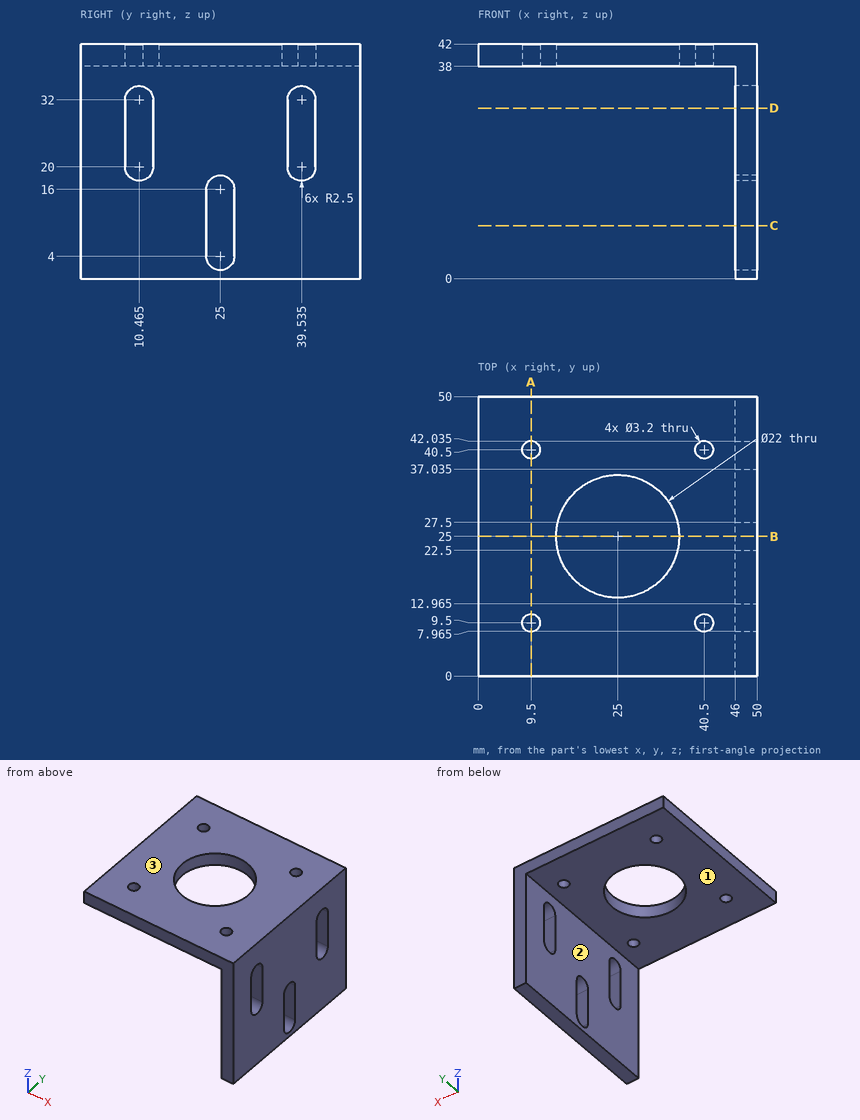
Source: three-view drawing plus pictorial views. Frame: mm from the lowest corner of the part. Coordinates: 2 decimals unless noted, no trailing zeros. Write each loop counter-clockwise with the first axis right and the second up, starting at its lowest first coordinate (ties: lowest second). Pieces come first, ordered by that corner, then holes. Notation, with made-up numbers: (77.5, 84.5) - (87.5, 84.5) arc R14 cw to (87.5, 104.5) - close; hole circle Ø9 at (-38.75, 57.25). An arc over 180 degrees is marked (long way). Return JSON: item names as keys, results as strings.
Item 1: Section query C-C (z = 9.5). Output: boundary loops of the cut face in (x, y), and give its area (3 significant figures).
Completed:
{"outline": "(46, 0) - (50, 0) - (50, 22.5) - (46, 22.5) - close; (46, 27.5) - (50, 27.5) - (50, 50) - (46, 50) - close", "area": "180 mm2"}
Item 2: Section query A-A (x = 9.5). Output: boundary loops of the cut face in (y, z), and give its area (3 significant figures).
Completed:
{"outline": "(0, 38) - (7.9, 38) - (7.9, 42) - (0, 42) - close; (11.1, 38) - (38.9, 38) - (38.9, 42) - (11.1, 42) - close; (42.1, 38) - (50, 38) - (50, 42) - (42.1, 42) - close", "area": "174 mm2"}
Item 3: Line query: L1, parallel to Y at x = 9.5, z = 39.8; L2, parallel to Y at x = 25, z = 39.8; L3, parallel to Y at x = 48, z = 6. Output: solid intervals per line, ascending.
Completed:
{"L1": "y = 0 to 7.9, 11.1 to 38.9, 42.1 to 50", "L2": "y = 0 to 14, 36 to 50", "L3": "y = 0 to 22.5, 27.5 to 50"}
Item 4: Pin query (flat end, axial travel): pin 1 Ø23 at (x, y) = (12, 19) entering from -Z; pin 2 Ø17.5 at (x, y) = (25, 25) entering from +Z; pin 3 Ø11.5 at (y, z) = (28.5, 15) entering from -X. Return the tip coordinate at first contact, or that it passes through.
Completed:
{"pin 1": "stops at z = 38", "pin 2": "passes through", "pin 3": "stops at x = 46"}
Item 5: Section query B-B (y = 25). Output: boundary loops of the cut face in (x, z), and give its area (3 significant figures).
Completed:
{"outline": "(0, 38) - (14, 38) - (14, 42) - (0, 42) - close; (36, 38) - (46, 38) - (46, 18.5) - (50, 18.5) - (50, 42) - (36, 42) - close; (46, 0) - (50, 0) - (50, 1.5) - (46, 1.5) - close", "area": "196 mm2"}
Item 6: Section query D-D (z = 30.5). Output: boundary loops of the cut face in (x, y) (3 decimals), and give its area (3 significant figures).
Completed:
{"outline": "(46, 0) - (50, 0) - (50, 7.965) - (46, 7.965) - close; (46, 12.965) - (50, 12.965) - (50, 37.035) - (46, 37.035) - close; (46, 42.035) - (50, 42.035) - (50, 50) - (46, 50) - close", "area": "160 mm2"}
Item 7: Pull-direction query (Z, two-part tool) for the marked faces 1, 2 and 3; classes: +Z half, -Z half, draft (parallel to the pull), parting line (faces both ways), or undercut.
Completed:
{"face 1": "-Z half", "face 2": "draft", "face 3": "+Z half"}
